The drawing under review shows one solid part. Ordinate dimensions are in mm from its lowest x, y, z. Coordinates: 2 decimals unless noted, no trailing zeros. Order: outer loops, then holes, each group sorted by start corner. A loop starts at its lowest first (then second) coordinate and runs counter-clockwise, first axis right, second up. Notation, with made-up numbers: (29, -22) -> (53, -22) arc R21 cw to (53, -7) -> close; hole circle Ø5 at (55, 67). An arc over 180 degrees is marked (long way). Use a Markdown table: item, result. Add a question column.
Q1. Add section A-A (y = 188). State the section outline as (x, z) points.
Q2. Add section B-B (x = 8.5). Count the separate pieces of the cut face and the enclosed holes in it, then the cut area to 3 significant figures.
Q3. Wall thickness on probe 1 along Y at (x, z) = (20.5, 13); probe 2 along Y at (x, z) = (15, 10.75); probe 3 along Z at (x, y) = (11.75, 12): over which ranges is each line inside the solid? List them lowest first.
Q4. Add section C-C (y = 150.5). State the section outline as (x, z) points, then the cut area to 3 significant figures.
Q5. Insertion check: pin 1 (3 mm diameter, centred on x = 9.5, y = 143, fed in from -Z); pin 2 (4 mm diameter, centred on y = 117.5, z = 8, fed in from -X); pin 3 (12 mm diameter, centred on x = 20.5, y = 79.5, fed in from +Z); pin 4 (4 mm diameter, centred on y = 12, z = 12.5, fed in from -X). Each pin has a flat end and moves straight along its axis. Give the tip position at first contact, or say it passes through.
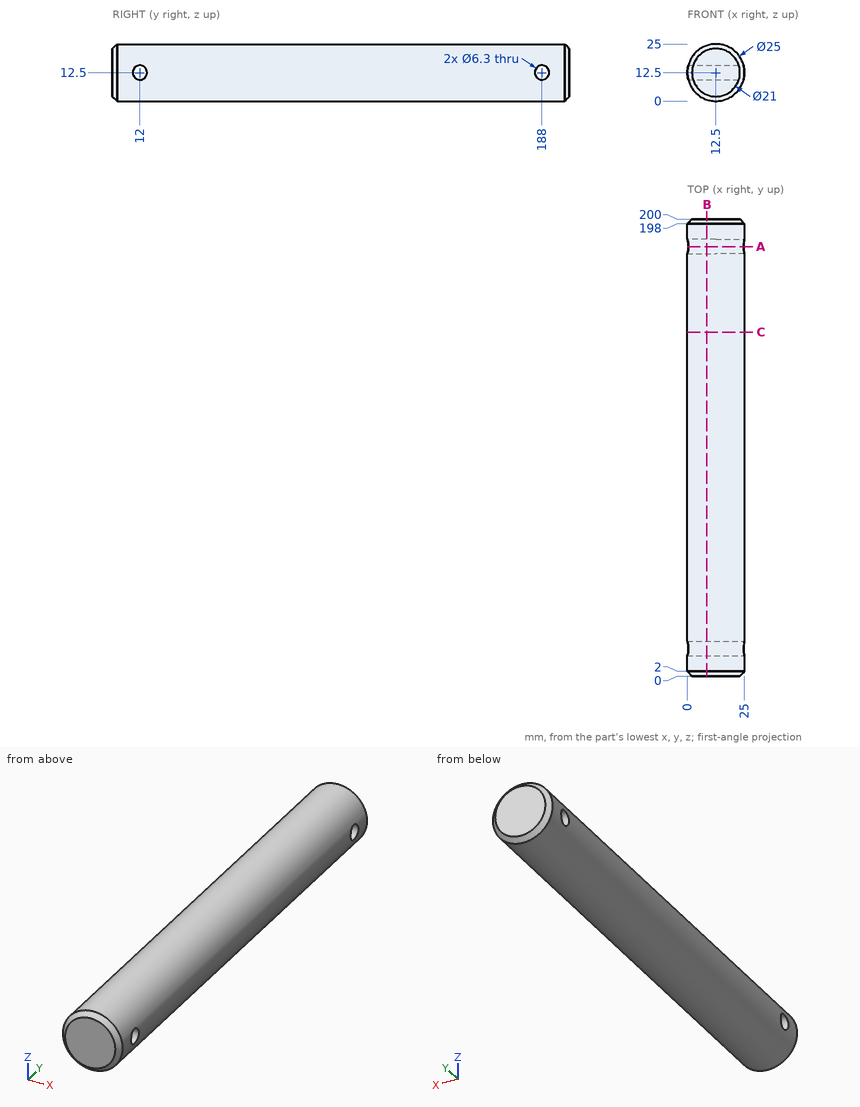
Established:
| question | item | result |
|---|---|---|
| 1 | outline | (0.4, 9.35) arc R12.5 ccw to (24.6, 9.35) -> close; (0.4, 15.65) -> (24.6, 15.65) arc R12.5 ccw to start |
| 2 | separate pieces | 1 |
| 2 | enclosed holes | 2 |
| 2 | area | 4,670 mm^2 |
| 3 | probe 1 | 0 to 8.89, 15.11 to 184.89, 191.11 to 200 |
| 3 | probe 2 | 0 to 9.38, 14.62 to 185.38, 190.62 to 200 |
| 3 | probe 3 | 0.02 to 9.35, 15.65 to 24.98 |
| 4 | outline | circle Ø25 at (12.5, 12.5) |
| 4 | area | 491 mm^2 |
| 5 | pin 1 | z = 0.09 |
| 5 | pin 2 | x = 0.25 |
| 5 | pin 3 | z = 24.84 |
| 5 | pin 4 | through |
